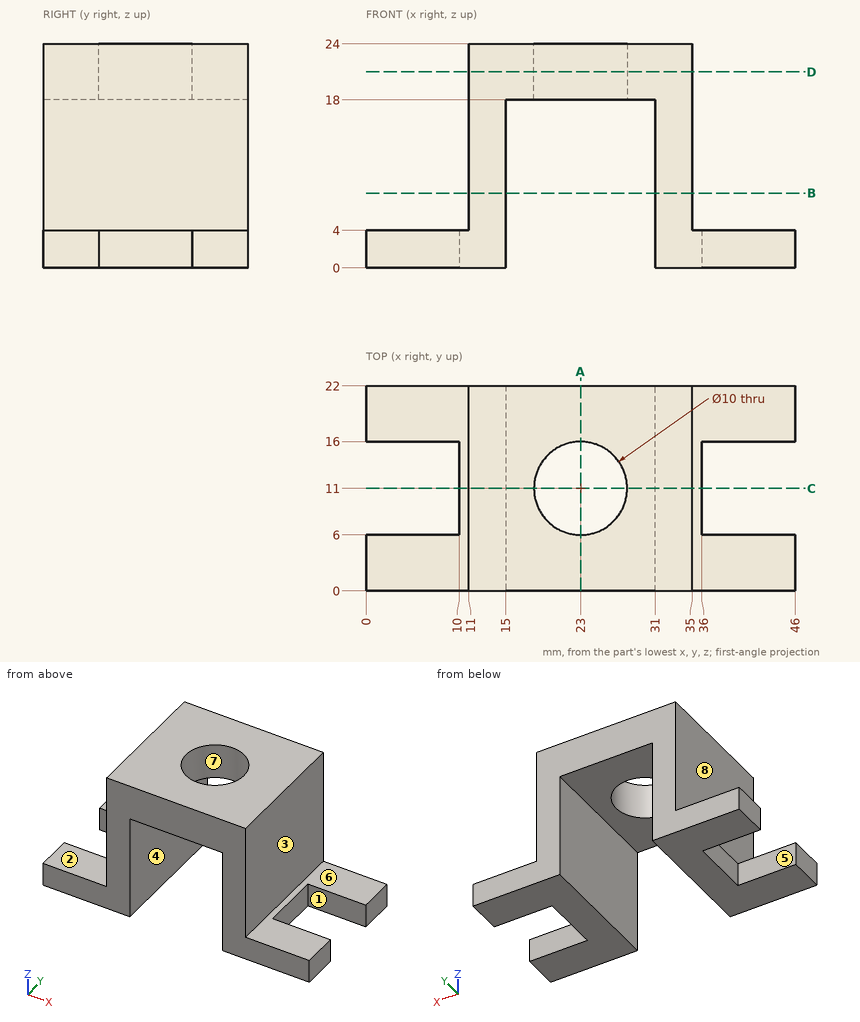
The drawing under review shows one solid part. Ordinate dimensions are in mm from its lowest x, y, z. A direction names the side the tool comes from. Round coordinates to 2 decimals unless told otherwise and drop trailing zeros. Loops run counter-clockwise (first coordinate to the right, second up) from the corner with the lowest first, then second, coordinate; pieces in that order, holes last. Notation, with made-up numbers: (-6.5, -20) -> (20.5, -20) arc R25 cw to (20.5, 10) -> close; hole circle Ø1 at (-26.75, 37). An arc over 180 degrees is marked (long way). Answer in a Markdown table with one row per item.
1) Consider section A-A, the plane x = 23. Write out the cut boundary in (y, z).
Taken from the geometry:
| item | result |
|---|---|
| outline | (0, 18) -> (6, 18) -> (6, 24) -> (0, 24) -> close; (16, 18) -> (22, 18) -> (22, 24) -> (16, 24) -> close |
2) Tool access review of the marked faces 1, 2, 3, 4 and 5: name each direction out of +Z, -Z, +X, -X, +Y, -Y from which nothing blocks a thin tool from reaching the whole face with its end or side.
Taken from the geometry:
| item | result |
|---|---|
| face 1 | +Z, -Z, +X |
| face 2 | +Z, -X, +Y, -Y |
| face 3 | +Z, +X, +Y, -Y |
| face 4 | -Z, +Y, -Y |
| face 5 | +Z, -Z, -X |
3) Wall thickness on line 1 along X through (y, z) = (4.5, 9.25); line 2 along Y through (x, z) = (23, 19.6); line 3 along Z through (x, y) = (36, 5): over which ranges is each line inside the solid? List them lowest first.
Taken from the geometry:
| item | result |
|---|---|
| line 1 | x = 11 to 15, 31 to 35 |
| line 2 | y = 0 to 6, 16 to 22 |
| line 3 | z = 0 to 4 |
4) Draft analysis for pull direction X (two halves, no side actions). For the marked faces 6, 7 and 8, state which applies: pulls with the +X half, pulls with the -X half, needs draft (parallel to the pull), parting line crosses it, or undercut.
Taken from the geometry:
| item | result |
|---|---|
| face 6 | needs draft |
| face 7 | undercut |
| face 8 | pulls with the -X half |
5) Consider section C-C, the plane y = 11. Write out the cut boundary in (x, z), plus the area to 3 significant figures.
Taken from the geometry:
| item | result |
|---|---|
| outline | (10, 0) -> (15, 0) -> (15, 18) -> (18, 18) -> (18, 24) -> (11, 24) -> (11, 4) -> (10, 4) -> close; (28, 18) -> (31, 18) -> (31, 0) -> (36, 0) -> (36, 4) -> (35, 4) -> (35, 24) -> (28, 24) -> close |
| area | 236 mm² |
6) Consider section D-D, the plane z = 21. Write out the cut boundary in (x, y).
Taken from the geometry:
| item | result |
|---|---|
| outline | (11, 0) -> (35, 0) -> (35, 22) -> (11, 22) -> close; hole circle Ø10 at (23, 11) |
7) Consider section B-B, the plane z = 8. Write out the cut boundary in (x, y), plus the area to 3 significant figures.
Taken from the geometry:
| item | result |
|---|---|
| outline | (11, 0) -> (15, 0) -> (15, 22) -> (11, 22) -> close; (31, 0) -> (35, 0) -> (35, 22) -> (31, 22) -> close |
| area | 176 mm² |
8) For pin 1 Ø2 at (y, z) = (7.5, 21.5) entering from -X; pin 2 Ø4 at (x, y) = (6, 8.5) entering from -Z; pin 3 Ø5.5 at (x, y) = (7.5, 12.5) entering from +Z; pin 4 Ø6 at (y, z) = (16, 11.5) entering from +X, all flat-tipped, find the tip position at first contact; note any pin that passes through.
Taken from the geometry:
| item | result |
|---|---|
| pin 1 | stops at x = 11 |
| pin 2 | passes through |
| pin 3 | stops at z = 4 |
| pin 4 | stops at x = 35 |
